Verification items for the finished model (mm, model axes). Face numbers are marked on the shaded views. Round coordinates to 2 decimals unless told otherwise and drop trailing zeros. Loops run counter-clockwise (first coordinate to the right, second up) from the corner with the lowest first, then second, coordinate; pieces in that order, holes last. Notation, with made-up numbers: M 5.25,27.5 L 17.25,27.5 A29 cw 17.25,61.5 Z; hole C -32,-25 d7. An arc over 180 degrees is marked long. Answer as CSV lines item,"result".
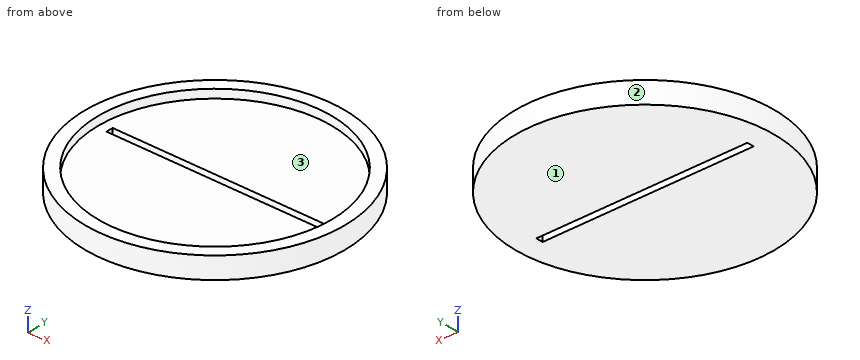
```python
from build123d import *

# Parameters (mm, degrees)
F0_R     = 15.24
F0_R_2   = 13.716
F1_DEPTH = 2.54
F0_W     = 25
F0_H     = 0.8382
F2_DEPTH = 1.524


with BuildPart() as f1:
    # F0 (on Top) → F1 (new body)
    with BuildSketch(Plane.XY):
        Circle(F0_R)
        Circle(F0_R_2, mode=Mode.SUBTRACT)
    extrude(amount=F1_DEPTH)

    # F0 (on Top) → F2 (join)
    with BuildSketch(Plane.XY):
        Circle(F0_R_2)
        Rectangle(F0_W, F0_H, mode=Mode.SUBTRACT)
    extrude(amount=F2_DEPTH)


solid = f1.part
```
1) Section check C-C (z = 0.95). Record the cut outline in (x, y), plus the area to 3 significant figures.
Here are the results:
outline,"C 0,0 d30.48; hole M -12.5,-0.42 L 12.5,-0.42 L 12.5,0.42 L -12.5,0.42 Z"
area,"709 mm^2"
2) Section check B-B (y = 0). Record the cut outline in (x, z).
Here are the results:
outline,"M -15.24,0 L -12.5,0 L -12.5,1.52 L -13.72,1.52 L -13.72,2.54 L -15.24,2.54 Z; M 12.5,0 L 15.24,0 L 15.24,2.54 L 13.72,2.54 L 13.72,1.52 L 12.5,1.52 Z"
3) Material ranges on probe 1 along Y at (x, z) = (0, 2.2); probe 2 along Z at (x, y) = (-4.5, -1); probe 3 along Y at (x, z) = (-6.5, 0.7), recorded low to high.
Here are the results:
probe 1,"y = -15.24 to -13.72, 13.72 to 15.24"
probe 2,"z = 0 to 1.52"
probe 3,"y = -13.78 to -0.42, 0.42 to 13.78"
4) Go/stop test with flat-tipped pins: pin 1 (6 mm diameter, centred on x = -1, y = -1, fed in from -Z); pin 2 (0.5 mm diameter, centred on x = 3.5, z = 0.5, fed in from +Y); pin 3 (0.5 mm diameter, centred on x = -1, z = 1, fed in from -Y). Record where each tip stops, or that it passes through.
Here are the results:
pin 1,"stops at z = 0"
pin 2,"stops at y = 14.89"
pin 3,"stops at y = -15.22"
5) Section check D-D (y = -6.5). Record the cut outline in (x, z), plus the area to 3 significant figures.
Here are the results:
outline,"M -13.78,0 L 13.78,0 L 13.78,2.54 L 12.08,2.54 L 12.08,1.52 L -12.08,1.52 L -12.08,2.54 L -13.78,2.54 Z"
area,"45.5 mm^2"
6) Section check A-A (x = 0). Record the cut outline in (y, z), plus the area to 3 significant figures.
Here are the results:
outline,"M -15.24,0 L -0.42,0 L -0.42,1.52 L -13.72,1.52 L -13.72,2.54 L -15.24,2.54 Z; M 0.42,0 L 15.24,0 L 15.24,2.54 L 13.72,2.54 L 13.72,1.52 L 0.42,1.52 Z"
area,"48.3 mm^2"
7) Draft check along Y on the marked faces 1, 2 and 3. Enter one of: +Y half, -Y half, draft (parallel to the pull), parting line (faces both ways), or undercut.
Here are the results:
face 1,"draft"
face 2,"parting line"
face 3,"undercut"
